from build123d import *

# Parameters (mm, degrees)
F0_R         = 3.5
F1_DEPTH     = 10
F0_R_2       = 2.75
F2_DEPTH     = 95
F3_DEPTH     = 90
F4_DEPTH     = 3
F5_T1_DEPTH  = 41
F5_T3_DEPTH  = 70
F5_T5_DEPTH  = 42
F5_T7_DEPTH  = 69
F5_T10_ANGLE = 90
F5_T12_ANGLE = 90
F5_T14_ANGLE = 90
F5_T16_ANGLE = 90
F0_R_3       = 2
F6_DEPTH     = 10
F7_DEPTH     = 5


# Not quite as in the source:
# - a fillet or chamfer that OpenCascade refuses, or shapes differently, is made with other operations: its cross-section is extruded or revolved along the edge and cut away or added


with BuildPart() as f1:
    # F0 (on Front) → F1 (new body)
    with BuildSketch(Plane.XZ):
        with BuildLine():
            Line((30.5, 29.5), (-30.5, 29.5))
            ThreePointArc((-30.5, 29.5), (-44.6421356237, 23.6421356237), (-50.5, 9.5))
            Line((-50.5, 9.5), (-50.5, -9.5))
            ThreePointArc((-50.5, -9.5), (-44.6421356237, -23.6421356237), (-30.5, -29.5))
            Line((-30.5, -29.5), (30.5, -29.5))
            ThreePointArc((30.5, -29.5), (44.6421356237, -23.6421356237), (50.5, -9.5))
            Line((50.5, -9.5), (50.5, 9.5))
            ThreePointArc((50.5, 9.5), (44.6421356237, 23.6421356237), (30.5, 29.5))
        make_face()
        with Locations((-46.59, 0)):
            Circle(F0_R, mode=Mode.SUBTRACT)
        with BuildLine():
            ThreePointArc((-40, 21), (-38.5355339059, 24.5355339059), (-35, 26))
            Line((-35, 26), (35, 26))
            ThreePointArc((35, 26), (38.5355339059, 24.5355339059), (40, 21))
            Line((40, 21), (40, -21))
            ThreePointArc((40, -21), (38.5355339059, -24.5355339059), (35, -26))
            Line((35, -26), (-35, -26))
            ThreePointArc((-35, -26), (-38.5355339059, -24.5355339059), (-40, -21))
            Line((-40, -21), (-40, 21))
        make_face(mode=Mode.SUBTRACT)
        with Locations((46.59, 0)):
            Circle(F0_R, mode=Mode.SUBTRACT)
    extrude(amount=F1_DEPTH)

    # F0 (on Front) → F2 (join)
    with BuildSketch(Plane.XZ):
        with BuildLine():
            Line((35, 26), (-35, 26))
            ThreePointArc((-35, 26), (-38.5355339059, 24.5355339059), (-40, 21))
            Line((-40, 21), (-40, -21))
            ThreePointArc((-40, -21), (-38.5355339059, -24.5355339059), (-35, -26))
            Line((-35, -26), (35, -26))
            ThreePointArc((35, -26), (38.5355339059, -24.5355339059), (40, -21))
            Line((40, -21), (40, 21))
            ThreePointArc((40, 21), (38.5355339059, 24.5355339059), (35, 26))
        make_face()
        with BuildLine():
            ThreePointArc((-37.5, 20.5), (-36.6213203436, 22.6213203436), (-34.5, 23.5))
            Line((-34.5, 23.5), (34.5, 23.5))
            ThreePointArc((34.5, 23.5), (36.6213203436, 22.6213203436), (37.5, 20.5))
            Line((37.5, 20.5), (37.5, -21.5))
            ThreePointArc((37.5, -21.5), (36.9142135624, -22.9142135624), (35.5, -23.5))
            Line((35.5, -23.5), (-34.5, -23.5))
            ThreePointArc((-34.5, -23.5), (-36.6213203436, -22.6213203436), (-37.5, -20.5))
            Line((-37.5, -20.5), (-37.5, 20.5))
        make_face(mode=Mode.SUBTRACT)
        with BuildLine():
            Line((34.5, 23.5), (-34.5, 23.5))
            ThreePointArc((-34.5, 23.5), (-36.6213203436, 22.6213203436), (-37.5, 20.5))
            Line((-37.5, 20.5), (-37.5, -20.5))
            ThreePointArc((-37.5, -20.5), (-36.6213203436, -22.6213203436), (-34.5, -23.5))
            Line((-34.5, -23.5), (35.5, -23.5))
            ThreePointArc((35.5, -23.5), (36.9142135624, -22.9142135624), (37.5, -21.5))
            Line((37.5, -21.5), (37.5, 20.5))
            ThreePointArc((37.5, 20.5), (36.6213203436, 22.6213203436), (34.5, 23.5))
        make_face()
        with Locations((-34.5, 20.5)):
            Circle(F0_R_2, mode=Mode.SUBTRACT)
        with Locations((34.5, 20.5)):
            Circle(F0_R_2, mode=Mode.SUBTRACT)
    extrude(amount=F2_DEPTH)

    # F0 (on Front) → F3 (cut)
    with BuildSketch(Plane.XZ):
        with BuildLine():
            Line((34.5, 23.5), (-34.5, 23.5))
            ThreePointArc((-34.5, 23.5), (-36.6213203436, 22.6213203436), (-37.5, 20.5))
            Line((-37.5, 20.5), (-37.5, -20.5))
            ThreePointArc((-37.5, -20.5), (-36.6213203436, -22.6213203436), (-34.5, -23.5))
            Line((-34.5, -23.5), (35.5, -23.5))
            ThreePointArc((35.5, -23.5), (36.9142135624, -22.9142135624), (37.5, -21.5))
            Line((37.5, -21.5), (37.5, 20.5))
            ThreePointArc((37.5, 20.5), (36.6213203436, 22.6213203436), (34.5, 23.5))
        make_face()
        with Locations((-34.5, 20.5)):
            Circle(F0_R_2, mode=Mode.SUBTRACT)
        with Locations((34.5, 20.5)):
            Circle(F0_R_2, mode=Mode.SUBTRACT)
    extrude(amount=F3_DEPTH, mode=Mode.SUBTRACT)

    # F0 (on Front) → F4 (join)
    with BuildSketch(Plane.XZ):
        with BuildLine():
            Line((35, 26), (-35, 26))
            ThreePointArc((-35, 26), (-38.5355339059, 24.5355339059), (-40, 21))
            Line((-40, 21), (-40, -21))
            ThreePointArc((-40, -21), (-38.5355339059, -24.5355339059), (-35, -26))
            Line((-35, -26), (35, -26))
            ThreePointArc((35, -26), (38.5355339059, -24.5355339059), (40, -21))
            Line((40, -21), (40, 21))
            ThreePointArc((40, 21), (38.5355339059, 24.5355339059), (35, 26))
        make_face()
        with BuildLine():
            ThreePointArc((-37.5, 20.5), (-36.6213203436, 22.6213203436), (-34.5, 23.5))
            Line((-34.5, 23.5), (34.5, 23.5))
            ThreePointArc((34.5, 23.5), (36.6213203436, 22.6213203436), (37.5, 20.5))
            Line((37.5, 20.5), (37.5, -21.5))
            ThreePointArc((37.5, -21.5), (36.9142135624, -22.9142135624), (35.5, -23.5))
            Line((35.5, -23.5), (-34.5, -23.5))
            ThreePointArc((-34.5, -23.5), (-36.6213203436, -22.6213203436), (-37.5, -20.5))
            Line((-37.5, -20.5), (-37.5, 20.5))
        make_face(mode=Mode.SUBTRACT)
    extrude(amount=-F4_DEPTH)

    # F5: fillet of radius 3 on 2 edges, made by hand

    # F5_s2 → F5_t1 (cut)
    with BuildSketch(Plane.XY.offset(-20.5)):
        with BuildLine():
            ThreePointArc((-40.5, 3), (-38.3786796564, 2.1213203436), (-37.5, 0))
            Line((-37.5, 0), (-37.5, 3))
            Line((-37.5, 3), (-40.5, 3))
        make_face()
    extrude(amount=F5_T1_DEPTH, mode=Mode.SUBTRACT)

    # F5_s4 → F5_t3 (cut)
    with BuildSketch(Plane.YZ.offset(-34.5)):
        with BuildLine():
            ThreePointArc((3, -26.5), (2.1213203436, -24.3786796564), (0, -23.5))
            Line((0, -23.5), (3, -23.5))
            Line((3, -23.5), (3, -26.5))
        make_face()
    extrude(amount=F5_T3_DEPTH, mode=Mode.SUBTRACT)

    # F5_s6 → F5_t5 (cut)
    with BuildSketch(Plane.XY.offset(-21.5)):
        with BuildLine():
            ThreePointArc((40.5, 3), (38.3786796564, 2.1213203436), (37.5, 0))
            Line((37.5, 0), (37.5, 3))
            Line((37.5, 3), (40.5, 3))
        make_face()
    extrude(amount=F5_T5_DEPTH, mode=Mode.SUBTRACT)

    # F5_s8 → F5_t7 (cut)
    with BuildSketch(Plane.YZ.offset(-34.5)):
        with BuildLine():
            ThreePointArc((3, 26.5), (2.1213203436, 24.3786796564), (0, 23.5))
            Line((0, 23.5), (3, 23.5))
            Line((3, 23.5), (3, 26.5))
        make_face()
    extrude(amount=F5_T7_DEPTH, mode=Mode.SUBTRACT)

    # F5_s9 → F5_t10 (revolve, cut)
    with BuildSketch(Plane.XY.offset(-21.5)):
        with BuildLine():
            ThreePointArc((40.5, 3), (38.3786796564, 2.1213203436), (37.5, 0))
            Line((37.5, 0), (37.5, 3))
            Line((37.5, 3), (40.5, 3))
        make_face()
    revolve(axis=Axis((35.5, 3, -21.5), (0, 1, 0)), revolution_arc=F5_T10_ANGLE, mode=Mode.SUBTRACT)

    # F5_s11 → F5_t12 (revolve, cut)
    with BuildSketch(Plane.YZ.offset(-34.5)):
        with BuildLine():
            ThreePointArc((3, -26.5), (2.1213203436, -24.3786796564), (0, -23.5))
            Line((0, -23.5), (3, -23.5))
            Line((3, -23.5), (3, -26.5))
        make_face()
    revolve(axis=Axis((-34.5, 3, -20.5), (0, 1, 0)), revolution_arc=F5_T12_ANGLE, mode=Mode.SUBTRACT)

    # F5_s13 → F5_t14 (revolve, cut)
    with BuildSketch(Plane.YZ.offset(34.5)):
        with BuildLine():
            ThreePointArc((0, 23.5), (2.1213203436, 24.3786796564), (3, 26.5))
            Line((3, 26.5), (3, 23.5))
            Line((3, 23.5), (0, 23.5))
        make_face()
    revolve(axis=Axis((34.5, 3, 20.5), (0, 1, 0)), revolution_arc=F5_T14_ANGLE, mode=Mode.SUBTRACT)

    # F5_s15 → F5_t16 (revolve, cut)
    with BuildSketch(Plane.XY.offset(20.5)):
        with BuildLine():
            ThreePointArc((-40.5, 3), (-38.3786796564, 2.1213203436), (-37.5, 0))
            Line((-37.5, 0), (-37.5, 3))
            Line((-37.5, 3), (-40.5, 3))
        make_face()
    revolve(axis=Axis((-34.5, 3, 20.5), (0, 1, 0)), revolution_arc=F5_T16_ANGLE, mode=Mode.SUBTRACT)

    # F0 (on Front) → F6 (join)
    with BuildSketch(Plane.XZ):
        with Locations((46.59, 0)):
            Circle(F0_R)
        with Locations((46.59, 0)):
            Circle(F0_R_3, mode=Mode.SUBTRACT)
        with Locations((-46.59, 0)):
            Circle(F0_R)
        with Locations((-46.59, 0)):
            Circle(F0_R_3, mode=Mode.SUBTRACT)
    extrude(amount=F6_DEPTH)

    # F0 (on Front) → F7 (cut)
    with BuildSketch(Plane.XZ):
        with Locations((46.59, 0)):
            Circle(F0_R)
        with Locations((46.59, 0)):
            Circle(F0_R_3, mode=Mode.SUBTRACT)
        with Locations((-46.59, 0)):
            Circle(F0_R)
        with Locations((-46.59, 0)):
            Circle(F0_R_3, mode=Mode.SUBTRACT)
    extrude(amount=F7_DEPTH, mode=Mode.SUBTRACT)


solid = f1.part
Design review of the part built by this model. Coordinates are the model's own, in mm. A direction names the side the tool comes from. Round coordinates to 2 decimals unless told otherwise and drop trailing zeros. Write each loop counter-clockwise with the first axis right and the second up, starting at its lowest first coordinate (ties: lowest second). Pieces come first, ordered by that corner, then holes.
Item 1: Consider section C-C on x = 46.59. Give the boundary of the cut face in (y, z).
Item 2: Draft analysis for pull direction Z (two halves, no side actions). For faces 1 (the flat face through (3.5, 0, 26.4)), 2 (the flat face through (0, -5, -29.5)), 3 (the cylindrical face through (-36.64, -45.63, 22.6)), state which applies: released by +Z, released by -Z, zero draft, split by the parting line, or undercut.
Item 3: Consider section D-D on z = -6. Give the boundary of the cut face in (x, y).
Item 4: For faces 4 (the cylindrical face through (36.6, -45.63, 22.64)), 5 (the cylindrical face through (-39, 1, -24)), 6 (the flat face through (0, 1, -26)), list the 3-axis set-ups (+Z, -Z, +X, -X, +Y, -Y) from which the entire face can be reached by the end or side of a thin tool; tool diameter is ignored.
Item 5: Wall thickness on L1, parallel to Z at x = 17, y = -7; L2, parallel to X at y = -92, z = 20; L3, parallel to Z at x = -30, y = -62.5: over which ranges is each line inside the solid? List them lowest first.
Item 6: Consider section B-B on y = -19.5. Give the boundary of the cut face in (x, z).
Item 7: Consider section A-A on z = 0. Count the separate pieces of the cut face and the enclosed holes in it, and give its area (3 significant figures).
Item 8: For pin 1 Ø12 at (y, z) = (-27, -20.5) entering from +X; pin 2 Ø12 at (x, y) = (-38, -52.5) entering from -Z; pin 3 Ø3.5 at (x, y) = (-10, 1.5) entering from +Z; pin 4 Ø17.5 at (x, z) = (-10.5, -8) entering from +Y, all flat-tipped, find the tip position at first contact; note any pin that passes through.
Check values:
1. outline: (-10, -21.38) - (0, -21.38) - (0, -3.5) - (-5, -3.5) - (-5, -2) - (-10, -2) - close; (-10, 2) - (-5, 2) - (-5, 3.5) - (0, 3.5) - (0, 21.38) - (-10, 21.38) - close
2. face 1: zero draft
2. face 2: released by -Z
2. face 3: undercut
3. outline: (-50.5, -10) - (-40, -10) - (-40, -95) - (40, -95) - (40, -10) - (50.5, -10) - (50.5, 0) - (40, 0) - (40, 2.96) arc R3 ccw to (37.5, 0) - (37.5, -90) - (-37.5, -90) - (-37.5, 0) arc R3 ccw to (-40, 2.96) - (-40, 0) - (-50.5, 0) - close
4. face 4: +Y
4. face 5: -Z, -X, +Y
4. face 6: -Z, +X, -X, +Y
5. L1: z = -29.5 to -23.5, 23.5 to 29.5
5. L2: x = -40 to -37.2, -31.8 to 31.8, 37.2 to 40
5. L3: z = -26 to -23.5, 23.5 to 26
6. outline: (-40, -21) arc R5 ccw to (-35, -26) - (35, -26) arc R5 ccw to (40, -21) - (40, 21) arc R5 ccw to (35, 26) - (-35, 26) arc R5 ccw to (-40, 21) - close; hole (-37.5, -20.5) arc R3 ccw to (-34.5, -23.5) - (35.5, -23.5) arc R2 ccw to (37.5, -21.5) - (37.5, 20.5) arc R3 ccw to (34.5, 23.5) - (-34.5, 23.5) arc R3 ccw to (-37.5, 20.5) - close
7. separate pieces: 3
7. enclosed holes: 0
7. area: 961 mm2
8. pin 1: stops at x = 40
8. pin 2: stops at z = -26
8. pin 3: stops at z = 29.5
8. pin 4: stops at y = -90
